```python
from build123d import *

# Parameters (mm, degrees)
SKETCH046_W            = 400
SKETCH046_H            = 60
PAD003_DEPTH           = 400
SKETCH047_W            = 412
SKETCH047_H            = 50
PAD010_DEPTH           = 406
SKETCH048_W            = 512
SKETCH048_H            = 912
PAD011_DEPTH           = 6
CUT001_PLACEMENT_ANGLE = 180


with BuildPart() as body002:
    # Sketch046 → Pad003 (new body, symmetric)
    with BuildSketch(Plane.XZ):
        with Locations((0, 30)):
            Rectangle(SKETCH046_W, SKETCH046_H)
    extrude(amount=PAD003_DEPTH, both=True)


with BuildPart() as cut001:
    # Sketch047 → Pad010 (new body, symmetric)
    with BuildSketch(Plane.XZ):
        with Locations((0, 25)):
            Rectangle(SKETCH047_W, SKETCH047_H)
    extrude(amount=PAD010_DEPTH, both=True)

    # Sketch048 (on Face3 of Pad010) → Pad011 (join)
    with BuildSketch(Plane(origin=(0, 0, 50), x_dir=(-1, 0, 0), z_dir=(0, 0, 1))):
        Rectangle(SKETCH048_W, SKETCH048_H)
    extrude(amount=PAD011_DEPTH)

    # Cut001: cut Body002
    add(body002.part, mode=Mode.SUBTRACT)


with BuildPart() as cut001_1:
    # Cut001 placement: moved
    add(cut001.part.rotate(Axis((0, 0, 0), (0, 1, 0)), CUT001_PLACEMENT_ANGLE))


solid = cut001_1.part
```
Geometry check sheet. Reference: the model listing, model coordinates, mm. A direction names the side the tool comes from. Give positions to 0.01 mm unless a question says otherwise; leave off trailing zeros. Order: outer loops, then holes, each group sorted by start corner. A loop starts at its lowest first (then second) coordinate and runs counter-clockwise, first axis right, second up.
1. Section check B-B, the plane y = 1. Enter the section's corners in (x, z), and give its area (3 significant figures).
2. Section check A-A, the plane z = -15. Enter the section's corners in (x, y), and give its area (3 significant figures).
3. Thickness scan on L1, parallel to Y at x = -17, z = -43; L2, parallel to X at y = 194.5, z = -13.5; L3, parallel to Z at x = 226.5, y = -122. Record the ranges inside material, lowest first.
4. Section check C-C, the plane x = 151. Enter the section's corners in (y, z).
5. Gauge pin test, flat ends, axial feed: pin 1 Ø17 at (x, z) = (76.5, -30) entering from -Y; pin 2 Ø5 at (x, z) = (-57.5, -16.5) entering from +Y; pin 3 Ø2 at (y, z) = (28.5, -34) entering from +X. Record the tip position at first contact, or that the pin passes through.
6. Section check D-D, the plane x = -220.5. Enter the section's corners in (y, z).
7. Access from +Z, -Z, +X, -X, +Y, -Y to the whole of each face (thin tool, end or side, straight path). Record for faces 4 (the face through (3, -406, -25)), 5 (the face through (-200, -6, -28)), 6 (the face through (206, -6, -25)).
8. Release check for a two-part mould opening along Y. For faces 1 (the face through (3, -400, -28)), 2 (the face through (3, 406, -25)), 3 (the face through (-206, -6, -25)) record: pulls with the +Y half, pulls with the -Y half, needs draft (parallel to the pull), parting line crosses it, or undercut.
Values follow:
1. outline: (-256, -56) - (-200, -56) - (-200, 0) - (-206, 0) - (-206, -50) - (-256, -50) - close; (200, -56) - (256, -56) - (256, -50) - (206, -50) - (206, 0) - (200, 0) - close
1. area: 1,270 mm2
2. outline: (-206, -406) - (206, -406) - (206, 406) - (-206, 406) - close; hole (-200, -400) - (200, -400) - (200, 400) - (-200, 400) - close
2. area: 14,500 mm2
3. L1: y = -406 to -400, 400 to 406
3. L2: x = -206 to -200, 200 to 206
3. L3: z = -56 to -50
4. outline: (-456, -56) - (-400, -56) - (-400, 0) - (-406, 0) - (-406, -50) - (-456, -50) - close; (400, -56) - (456, -56) - (456, -50) - (406, -50) - (406, 0) - (400, 0) - close
5. pin 1: stops at y = -406
5. pin 2: stops at y = 406
5. pin 3: stops at x = 206
6. outline: (-456, -56) - (456, -56) - (456, -50) - (-456, -50) - close
7. face 4: +Z, +X, -X, -Y
7. face 5: +Z, -Z
7. face 6: +Z, +X, +Y, -Y
8. face 1: undercut
8. face 2: pulls with the +Y half
8. face 3: needs draft
